```python
from build123d import *

# Parameters (mm, degrees)
F0_R     = 17.5
F1_DEPTH = 11
F3_R     = 15
F5_R     = 3.175
F6_DEPTH = 26.001


with BuildPart() as f1:
    # F0 (on Right) → F1 (new body, symmetric)
    with BuildSketch(Plane.YZ):
        Circle(F0_R)
    extrude(amount=F1_DEPTH, both=True)

    # F4: sweep along a path in F2
    with BuildLine(Plane.YZ) as f4_path:
        CenterArc((0, 0), 28, 0, 360)
    # F3 (on Front) → F4 (sweep)
    with BuildSketch(Plane.XZ):
        with Locations((0, -28)):
            Circle(F3_R)
    sweep(path=f4_path.line)

    # F5 (on face) → F6 (cut, through all)
    with BuildSketch(Plane.YZ.offset(11)):
        Circle(F5_R)
    extrude(amount=-F6_DEPTH, mode=Mode.SUBTRACT)


solid = f1.part
```
The model under review builds one solid part; all positions refer to its coordinate system, in mm. A direction names the side the tool comes from. Round coordinates to 2 decimals unless told otherwise and drop trailing zeros. Loops run counter-clockwise (first coordinate to the right, second up) from the corner with the lowest first, then second, coordinate; pieces in that order, holes last. Notation, with made-up numbers: M 45.25,14.5 L 86.25,14.5 A25 cw 86.25,32.5 Z; hole C -23,54.25 d3. An arc over 180 degrees is marked long. Put each result on its own line as item: value.
Q1. Consider section A-A, the plane y = 0. Give the boundary of the cut face in (x, z) (3 decimals), then the cut area to 3 significant figures.
Result set:
outline: M -11,-17.5 L -10.712,-17.5 A15 ccw long 10.712,-17.5 L 11,-17.5 L 11,-3.175 L -11,-3.175 Z; M -11,3.175 L 11,3.175 L 11,17.5 L 10.712,17.5 A15 ccw long -10.712,17.5 L -11,17.5 Z
area: 1,910 mm²
Q2. Consider section C-C, the plane x = 9. Give the boundary of the cut face in (y, z) (3 decimals), then the cut area to 3 significant figures.
Result set:
outline: C 0,0 d80; hole C 0,0 d6.35
area: 4,990 mm²
Q3. For pin 1 (6 mm diameter, centred on x = -6, y = -7.5, fed in from +Z); pin 2 (3 mm diameter, centred on x = -5.5, z = 9.5, fed in from +Y); pin 3 (10 mm diameter, centred on y = 0, z = -5.5, fed in from +X); pin 4 (10 mm diameter, centred on y = -7, z = 22.5, fed in from +X), all flat-tipped, find the tip position at first contact; note any pin that passes through.
Result set:
pin 1: stops at z = 42.18
pin 2: stops at y = 41.49
pin 3: stops at x = 11
pin 4: stops at x = 15
Q4. To check wall thickness, follow L1, parallel to Z at x = 0, y = 0 (3 decimals); L2, parallel to X at y = 6.5, z = 5.5; L3, parallel to Z at x = 4, y = 0 (3 decimals). State the ranges of each line that lie inside material, in increasing order.
Result set:
L1: z = -43 to -3.175, 3.175 to 43
L2: x = -11 to 11
L3: z = -42.457 to -3.175, 3.175 to 42.457
Q5. Consider section D-D, the plane x = -6. Give the boundary of the cut face in (y, z) (3 decimals), then the cut area to 3 significant figures.
Result set:
outline: C 0,0 d83.495; hole C 0,0 d6.35
area: 5,440 mm²
Q6. Machinability: for faces 1 (the cylindrical face through (0.15, -0.69, -3.1)), 2 (the flat face through (11, 0, -4)), 3 (the flat face through (-11, 0, -4)), which of the approach directions +Z, -Z, +X, -X, +Y, -Y give a long, thin tool a straight path to every point of the face, cutting with its end or side? Answer none if there is none.
Result set:
face 1: +X, -X
face 2: +X
face 3: -X
